Model file for the job. Use its own axes, mm. Coordinates: 2 decimals unless noted, no trailing zeros. Order: outer loops, then holes, each group sorted by start corner. A loop starts at its lowest first (then second) coordinate and runs counter-clockwise, first axis right, second up. Notation, with made-up numbers: M -1.75,55 L 41.25,55 A10 ccw 41.25,62 Z; hole C -11.5,64.5 d1. An arc over 180 degrees is marked long. Return JSON: item names as keys, results as strings.
```python
from build123d import *

# Parameters (mm, degrees)
PAD004_DEPTH         = 3
SKETCH053_R          = 1.7
POCKET024_DEPTH      = 0.001
POCKET024_DEPTH_BACK = 3.001


with BuildPart() as part:
    # Sketch052 → Pad004 (new body)
    with BuildSketch(Plane.XY):
        with BuildLine():
            ThreePointArc((276.917507, 200.990417), (155.4148, 304.8388), (0, 342.170212))
            Line((0, 327.170212), (0, 342.170212))
            ThreePointArc((263.979122, 193.275376), (147.9973, 291.782704), (0, 327.170212))
            ThreePointArc((263.979122, 193.275376), (264.57986, 192.887597), (265.285977, 193.000099))
            Line((265.285977, 193.000099), (276.60821, 199.536993))
            ThreePointArc((276.60821, 199.536993), (277.086308, 200.194873), (276.917507, 200.990417))
        make_face()
    pad004 = extrude(amount=PAD004_DEPTH)

    # Mirrored009: Pad004 across Sketch052 V_Axis
    add(pad004.mirror(Plane(origin=(0, 0, 0), x_dir=(0, 0, 1), z_dir=(1, 0, 0))))

    # Sketch053 → Pocket024 (cut, two sides)
    with BuildSketch(Plane.XY) as pocket024_sk:
        with Locations((99.631602, 319.496001)):
            Circle(SKETCH053_R)
        with Locations((265.05233, 204.331625)):
            Circle(SKETCH053_R)
        with Locations((-99.631602, 319.496001)):
            Circle(SKETCH053_R)
        with Locations((-265.05233, 204.331625)):
            Circle(SKETCH053_R)
    extrude(amount=-POCKET024_DEPTH, mode=Mode.SUBTRACT)
    extrude(pocket024_sk.sketch, amount=POCKET024_DEPTH_BACK, mode=Mode.SUBTRACT)


solid = part.part
```
Item 1: Wall check: line 1 (X direction, y = 204.5, z = 0.4); line 2 (X direction, y = 232, z = 1.9); line 3 (X direction, y = 260, z = 1.9). Give the ranges that are in metal, low to high.
Check result:
{"line 1": "x = -274.34 to -266.74, -263.36 to -255.38, 255.38 to 263.36, 266.74 to 274.34", "line 2": "x = -251.51 to -230.69, 230.69 to 251.51", "line 3": "x = -222.44 to -198.6, 198.6 to 222.44"}
Item 2: Saw through at A-A (y = 290.5). Write the cut outline in (x, z).
Check result:
{"outline": "M -180.8,0 L -150.5,0 L -150.5,3 L -180.8,3 Z; M 150.5,0 L 180.8,0 L 180.8,3 L 150.5,3 Z"}
Item 3: Saw through at D-D (x = 183). Write the cut outline in (y, z), and give its area (3 significant figures).
Check result:
{"outline": "M 271.2,0 L 289.12,0 L 289.12,3 L 271.2,3 Z", "area": "53.8 mm2"}
Item 4: Drop flat-ended pins along their axis: pin 1 Ø5.5 at (x, y) = (-99.63, 319.5) entering from +Z; pin 2 Ø1.5 at (y, z) = (316.5, 0.5) entering from -X. Give the stop position or say it passes through.
Check result:
{"pin 1": "stops at z = 3", "pin 2": "stops at x = -131.84"}
Item 5: Saw through at C-C (y = 262). Write the cut outline in (x, z), and give its area (3 significant figures).
Check result:
{"outline": "M -220.08,0 L -195.95,0 L -195.95,3 L -220.08,3 Z; M 195.95,0 L 220.08,0 L 220.08,3 L 195.95,3 Z", "area": "145 mm2"}
Item 6: Saw through at B-B (z = 1.65). Write the cut outline in (x, y), and give its area (3 significant figures).
Check result:
{"outline": "M -276.92,200.99 A1 ccw -276.61,199.54 L -265.29,193 A1 ccw -263.98,193.28 A327.17 cw 0,327.17 A327.17 cw 263.98,193.28 A1 ccw 265.29,193 L 276.61,199.54 A1 ccw 276.92,200.99 A342.17 ccw 0,342.17 A342.17 ccw Z; hole C -265.05,204.33 d3.4; hole C -99.63,319.5 d3.4; hole C 99.63,319.5 d3.4; hole C 265.05,204.33 d3.4", "area": "9,440 mm2"}
